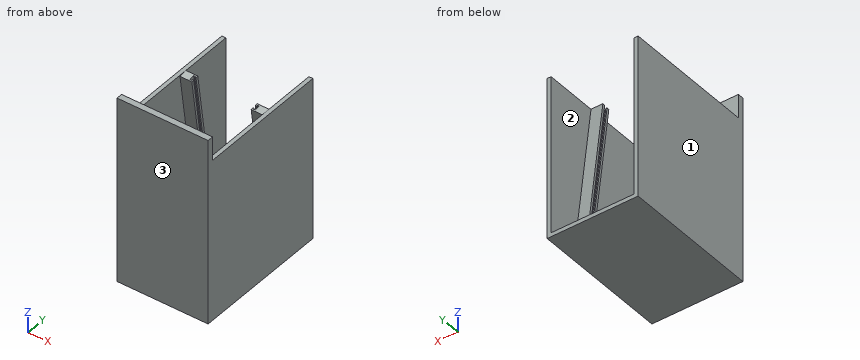
from build123d import *

# Parameters (mm, degrees)
SKETCH1_W           = 292.1
SKETCH1_H           = 596.9
BOSS_EXTRUDE1_DEPTH = 19.05
BOSS_EXTRUDE2_DEPTH = 425.45
BOSS_EXTRUDE3_DEPTH = 38.1
CUT_EXTRUDE1_DEPTH  = 10.16
CUT_EXTRUDE2_START  = -3.175
SKETCH5_W           = 6.35
SKETCH5_H           = 479.722786497
CUT_EXTRUDE2_DEPTH  = 16.51
SKETCH6_W           = 25.4
SKETCH6_H           = 177.8
BOSS_EXTRUDE4_DEPTH = 241.3
BOSS_EXTRUDE6_DEPTH = 38.1
CUT_EXTRUDE3_DEPTH  = 3.81


with BuildPart() as part:
    # Sketch1 → Boss-Extrude1 (new body)
    with BuildSketch(Plane(origin=(0, 0, 0), x_dir=(1, 0, 0), z_dir=(0, 1, 0))):
        Rectangle(SKETCH1_W, SKETCH1_H)
    extrude(amount=BOSS_EXTRUDE1_DEPTH)

    # Sketch2 → Boss-Extrude2 (add)
    with BuildSketch(Plane(origin=(0, 19.05, 0), x_dir=(1, 0, 0), z_dir=(0, 1, 0))):
        Polygon((-146.05, -222.25), (-146.05, 298.45), (146.05, 298.45), (146.05, -222.25), (133.35, -222.25), (133.35, 285.75), (-133.35, 285.75), (-133.35, -222.25), align=None)
    extrude(amount=BOSS_EXTRUDE2_DEPTH)

    # Sketch3 → Boss-Extrude3 (add)
    with BuildSketch(Plane(origin=(-133.35, 0, 0), x_dir=(0, 0, -1), z_dir=(1, 0, 0))):
        Polygon((-222.25, 275.074993173), (260.35, 342.9), (263.884996764, 317.747191054), (-218.715003236, 249.922184227), align=None)
    boss_extrude3 = extrude(amount=BOSS_EXTRUDE3_DEPTH)

    # Sketch4 → Cut-Extrude1 (cut)
    with BuildSketch(Plane(origin=(-95.25, 0, 0), x_dir=(0, 0, -1), z_dir=(1, 0, 0))):
        Polygon((-221.196449058, 267.5785887), (-219.768554178, 257.4185887), (255.285603139, 324.183096498), (253.857708258, 334.343096498), align=None)
    cut_extrude1 = extrude(amount=-CUT_EXTRUDE1_DEPTH, mode=Mode.SUBTRACT)

    # Sketch5 → Cut-Extrude2 (cut)
    with BuildSketch(Plane(origin=(0, 292.880820502, 41.161714982), x_dir=(1, 0, 0), z_dir=(0, -0.9902680687415715, -0.13917310096005858)).offset(CUT_EXTRUDE2_START)):
        with Locations((-102.235, -58.057354767)):
            Rectangle(SKETCH5_W, SKETCH5_H)
    cut_extrude2 = extrude(amount=CUT_EXTRUDE2_DEPTH, mode=Mode.SUBTRACT)

    # Mirror1: Boss-Extrude3, Cut-Extrude1, Cut-Extrude2 across plane
    add(boss_extrude3.mirror(Plane(origin=(0, 0, 0), x_dir=(0, 0, 1), z_dir=(1, 0, 0))))
    add(cut_extrude1.mirror(Plane(origin=(0, 0, 0), x_dir=(0, 0, 1), z_dir=(1, 0, 0))), mode=Mode.SUBTRACT)
    add(cut_extrude2.mirror(Plane(origin=(0, 0, 0), x_dir=(0, 0, 1), z_dir=(1, 0, 0))), mode=Mode.SUBTRACT)

    # Sketch6 → Boss-Extrude4 (add)
    with BuildSketch(Plane(origin=(0, 19.05, 0), x_dir=(1, 0, 0), z_dir=(0, 1, 0))):
        with Locations((0, 196.85)):
            Rectangle(SKETCH6_W, SKETCH6_H)
    extrude(amount=BOSS_EXTRUDE4_DEPTH)

    # Sketch8 → Boss-Extrude6 (add)
    with BuildSketch(Plane.XY.offset(-285.75)):
        with BuildLine():
            Line((-123.19, 19.05), (-41.91, 19.05))
            ThreePointArc((-41.91, 19.05), (-34.725795103, 22.025795103), (-31.75, 29.21))
            Line((-31.75, 29.21), (-31.75, 148.59))
            ThreePointArc((-31.75, 148.59), (-34.725795103, 155.774204897), (-41.91, 158.75))
            Line((-41.91, 158.75), (-123.19, 158.75))
            ThreePointArc((-123.19, 158.75), (-130.374204897, 155.774204897), (-133.35, 148.59))
            Line((-133.35, 148.59), (-133.35, 29.21))
            ThreePointArc((-133.35, 29.21), (-130.374204897, 22.025795103), (-123.19, 19.05))
        make_face()
    extrude(amount=BOSS_EXTRUDE6_DEPTH)

    # Sketch9 → Cut-Extrude3 (cut)
    with BuildSketch(Plane.XY.offset(-247.65)):
        with BuildLine():
            Line((-118.11, 139.7), (-46.99, 139.7))
            ThreePointArc((-46.99, 139.7), (-45.193948776, 138.956051224), (-44.45, 137.16))
            Line((-44.45, 137.16), (-44.45, 66.04))
            ThreePointArc((-44.45, 66.04), (-45.193948776, 64.243948776), (-46.99, 63.5))
            Line((-46.99, 63.5), (-118.11, 63.5))
            ThreePointArc((-118.11, 63.5), (-119.906051224, 64.243948776), (-120.65, 66.04))
            Line((-120.65, 66.04), (-120.65, 137.16))
            ThreePointArc((-120.65, 137.16), (-119.906051224, 138.956051224), (-118.11, 139.7))
        make_face()
    extrude(amount=-CUT_EXTRUDE3_DEPTH, mode=Mode.SUBTRACT)


solid = part.part
CAD build for the part. Positions are in the model's coordinates, mm. Face numbers are marked on the shaded views. Give positions to 0.01 mm unless a question says otherwise; leave off trailing zeros. Order: outer loops, then holes, each group sorted by start corner. A loop starts at its lowest first (then second) coordinate and runs counter-clockwise, first axis right, second up. Notation, with made-up numbers: (-9, 34.5) -> (14, 34.5) arc R22 ccw to (14, 55.5) -> close; hole circle Ø1 at (-11.5, -6). An arc over 180 degrees is marked (long way). Return JSON: item names as keys, results as strings.
Q1. Mould opens along Y. For the marked faces 1, 2 and 3 say: pulls with the +Y half, pulls with the -Y half, needs draft (parallel to the pull), parting line crosses it, or undercut.
Working result:
{"face 1": "needs draft", "face 2": "undercut", "face 3": "pulls with the -Y half"}
Q2. Flat gauge pins, fed straight in: pin 1 (1 mm diameter, centred on x = -55.5, y = 193.5, fed in from +Z); pin 2 (19 mm diameter, centred on x = -62.5, z = -262.5, fed in from +Y); pin 3 (4 mm diameter, centred on x = -139.5, y = 189.5, fed in from +Z). Where does each tip first touch, or does it go through?
Working result:
{"pin 1": "z = -285.75", "pin 2": "y = 158.75", "pin 3": "z = 222.25"}
Q3. Saw through at C-C (z = 253). Write the cut outline in (x, y).
Working result:
{"outline": "(-146.05, 0) -> (146.05, 0) -> (146.05, 19.05) -> (-146.05, 19.05) -> close"}
Q4. Saw through at A-A (x = -71). Write the cut outline in (y, z), then the cut area to 3 significant figures.
Working result:
{"outline": "(0, -298.45) -> (444.5, -298.45) -> (444.5, -285.75) -> (158.75, -285.75) -> (158.75, -247.65) -> (139.7, -247.65) -> (139.7, -251.46) -> (63.5, -251.46) -> (63.5, -247.65) -> (19.05, -247.65) -> (19.05, 298.45) -> (0, 298.45) -> close", "area": "21,800 mm²"}
Q5. Saw through at B-B (y = 357.5). Write the cut outline in (x, z).
Working result:
{"outline": "(-146.05, -298.45) -> (146.05, -298.45) -> (146.05, 222.25) -> (133.35, 222.25) -> (133.35, -285.75) -> (-133.35, -285.75) -> (-133.35, 222.25) -> (-146.05, 222.25) -> close"}
Q6. Drill centre lines: line 1 (X direction, y = 116.5, z = -124); line 2 (X direction, y = 36.5, z = -265.5); line 3 (Y direction, x = -100, z = -226.5). Where is each one in solid material? Low to high.
Working result:
{"line 1": "-146.05 to -133.35, -12.7 to 12.7, 133.35 to 146.05", "line 2": "-146.05 to -31.75, -12.7 to 12.7, 133.35 to 146.05", "line 3": "0 to 19.05, 312.49 to 317.03, 333.7 to 338.14"}
Q7. Saw through at D-D (y = 89.5). Write the cut outline in (x, z).
Working result:
{"outline": "(-146.05, -298.45) -> (146.05, -298.45) -> (146.05, 222.25) -> (133.35, 222.25) -> (133.35, -285.75) -> (12.7, -285.75) -> (12.7, -107.95) -> (-12.7, -107.95) -> (-12.7, -285.75) -> (-31.75, -285.75) -> (-31.75, -247.65) -> (-44.45, -247.65) -> (-44.45, -251.46) -> (-120.65, -251.46) -> (-120.65, -247.65) -> (-133.35, -247.65) -> (-133.35, 222.25) -> (-146.05, 222.25) -> close"}
